The listing builds one solid part. Answer for the finished solid, in the listing's coordinates (mm). Face numbers are marked on the shaded views. A direction names the side the tool comes from. Round coordinates to 2 decimals unless told otherwise and drop trailing zeros. Write each loop counter-clockwise with the first axis right and the second up, starting at its lowest first coordinate (ties: lowest second). Pieces come first, ordered by that corner, then holes.
(1) A cutting plane is placed at B-B, the plane y = -45. Give the vertices of the cut face in (x, z), and give its area (3 significant figures).
(2) A cutting plane is placed at A-A, the plane y = -21.5. Give the vertices of the cut face in (x, z), and give its area (3 significant figures).
(3) For the marked faces 3 and 4, determine the directions among +Z, -Z, +X, -X, +Y, -Y from which every point of the face is accessible in a straight line to the end or side of a thin tool.
(4) Each of these flat-tipped pins is pushed along its axis until it touches: pin 1 Ø12 at (x, y) = (5.5, -26) entering from +Z; pin 2 Ø5 at (y, z) = (-21.5, -8) entering from +X; pin 3 Ø1.5 at (y, z) = (-33, -1) entering from +X. Where does it stop, or does it pass through?
(5) Find the intervals of material crossed by probe 1 along Z at (x, y) = (-0.25, -7); probe 2 along Z at (x, y) = (1.5, -28); probe 3 along X at (y, z) = (14, -0.25), in increasing order.
(6) The mould has two halves that part along X. Classify the marked faces 1 and 2: +X half, -X half, draft (parallel to the pull), parting line (faces both ways), or undercut.
from build123d import *

# Parameters (mm, degrees)
F0_R     = 9.385
F1_DEPTH = 52.8
F1_TAPER = 2.5
F2_R     = 9.4
F3_DEPTH = 18.8
F4_R     = 9.4
F5_DEPTH = 20.4
F5_TAPER = 1


with BuildPart() as f1:
    # F0 (on Front) → F1 (new body)
    with BuildSketch(Plane.XZ):
        Circle(F0_R)
    extrude(amount=F1_DEPTH, taper=F1_TAPER)

    # F2 (on face) → F3 (join)
    with BuildSketch(Plane(origin=(0, 0, 0), x_dir=(-1, 0, 0), z_dir=(0, 1, 0))):
        Circle(F2_R)
    extrude(amount=F3_DEPTH)

    # F4 (on face) → F5 (join)
    with BuildSketch(Plane(origin=(0, 18.8, 0), x_dir=(-1, 0, 0), z_dir=(0, 1, 0))):
        Circle(F4_R)
    extrude(amount=F5_DEPTH, taper=F5_TAPER)

    # F6 (on Top) → F7 (revolve)
    with BuildSketch(Plane.XY):
        Polygon((-8.708294537, -14.1886593821), (-9.2448791865, -1.5), (-10.3712912667, -3.2655011038), align=None)
    revolve(axis=Axis((0, -52.8, 0), (0, 1, 0)))


solid = f1.part
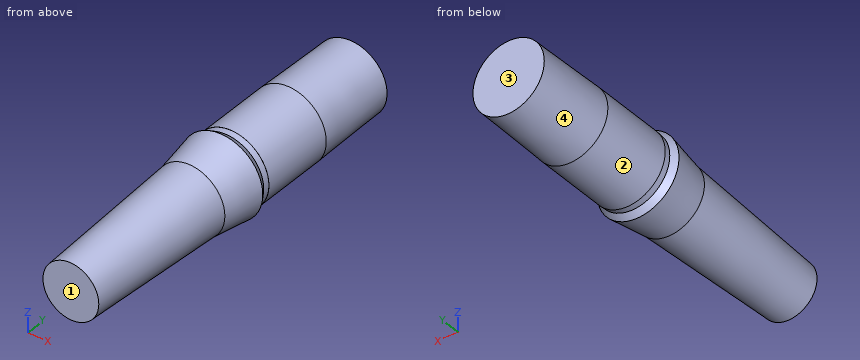
Solutions:
1. outline: circle Ø14.84 at (0, 0)
1. area: 173 mm2
2. outline: circle Ø16.89 at (0, 0)
2. area: 224 mm2
3. face 3: +Z, -Z, +X, -X, +Y
3. face 4: +Y
4. pin 1: stops at z = 8.38
4. pin 2: stops at x = 6.41
4. pin 3: stops at x = 7.95
5. probe 1: z = -9.8 to 9.8
5. probe 2: z = -8.02 to 8.02
5. probe 3: x = -9.4 to 9.4
6. face 1: draft
6. face 2: parting line
